For this review, take the finished solid that the model builds, in its own axes (mm). A direction names the side the tool comes from. Round coordinates to 2 decimals unless told otherwise and drop trailing zeros. Write each loop counter-clockwise with the first axis right and the second up, starting at its lowest first coordinate (ties: lowest second). Pieces come first, ordered by that corner, then holes. Notation, with made-up numbers: (-25.5, 6) - (-8.5, 6) arc R28 cw to (-8.5, 33) - close; hole circle Ø3 at (-37.5, 26.25). An arc over 180 degrees is marked (long way). One line per item, written item: value. Start each with the question number.
Q1. Add section A-A on y = 0. Write out the cut boundary in (x, z), and give its area (3 significant figures).
Q2. Mouldability with a two-part tool opening along Z and no side actions: class faces 4 (the face through (24.12, 0.03, 14.66)), 5 (the face through (22.146, 0.12, 50.945)), 6 (the face through (26.2, 0, -17.848)) as +Z half, -Z half, draft (parallel to the pull), parting line (faces both ways), or undercut.
Q3. For probe 1 along Z at (x, y) = (23.25, -2.25); probe 2 along Y at (x, z) = (25, 25); probe 3 along Z at (x, y) = (26.25, 1.25), list the stretches that pass through material, from the lowest coordinate up.
Q4. Tool access review of faces 1 (the face through (23.744, 0.049, -22.918)), 2 (the face through (21.12, 0.16, 55.23)), 3 (the face through (27, 2, 54.494)): name each direction out of +Z, -Z, +X, -X, +Y, -Y from which nothing blocks a thin tool from reaching the whole face with its end or side.
Q5. Add section B-B on z = -0.5. Write out the cut boundary in (x, y).
Q6. Clearance check with flat-ended pins moving along their axes: pin 1 Ø3 at (y, z) = (-2.5, 26) entering from +X; pin 2 Ø3 at (x, z) = (27, 13) entering from +Y. State where each tip first meets the part, or that it passes through.
```python
from build123d import *

# Parameters (mm, degrees)
SKETCH3_R          = 0.75
CUT_EXTRUDE6_DEPTH = 84.84194368


with BuildPart() as part:
    # Sketch2 → Revolve4 (revolve)
    with BuildSketch(Plane(origin=(0, 0, 0), x_dir=(1, 0, 0), z_dir=(0, 1, 0))):
        Polygon((24.868249983, 17.00561082), (24.868249983, -55.99438918), (28.618249983, -55.99438918), (28.618249983, -54.49438918), (27.593249983, -54.49438918), (27.593249983, -47.49438918), (27.968249983, -47.49438918), (27.968249983, 17.8475545), (25.993249983, 17.8475545), (25.993249983, 27.8475545), (24.868249983, 27.8475545), align=None)
    revolve(axis=Axis((24.868249983, 0, -17.00561082), (0, 0, 1)))

    # Sketch3 → Cut-Extrude6 (cut, through all)
    with BuildSketch(Plane.XY.offset(55.99438918)):
        with Locations((24.868249983, 0)):
            Circle(SKETCH3_R)
    extrude(amount=-CUT_EXTRUDE6_DEPTH, mode=Mode.SUBTRACT)


solid = part.part
```
Result set:
1. outline: (21.12, 54.49) - (22.14, 54.49) - (22.14, 47.49) - (21.77, 47.49) - (21.77, -17.85) - (23.74, -17.85) - (23.74, -27.85) - (24.12, -27.85) - (24.12, 55.99) - (21.12, 55.99) - close; (25.62, -27.85) - (25.99, -27.85) - (25.99, -17.85) - (27.97, -17.85) - (27.97, 47.49) - (27.59, 47.49) - (27.59, 54.49) - (28.62, 54.49) - (28.62, 55.99) - (25.62, 55.99) - close
1. area: 351 mm^2
2. face 4: draft
2. face 5: undercut
2. face 6: -Z half
3. probe 1: z = -17.85 to 47.49, 54.49 to 55.99
3. probe 2: y = -3.1 to -0.74, 0.74 to 3.1
3. probe 3: z = -17.85 to 55.99
4. face 1: -Z
4. face 2: +Z, -Z
4. face 3: none
5. outline: circle Ø6.2 at (24.87, 0); hole circle Ø1.5 at (24.87, 0)
6. pin 1: stops at x = 27.8
6. pin 2: stops at y = 3.03
